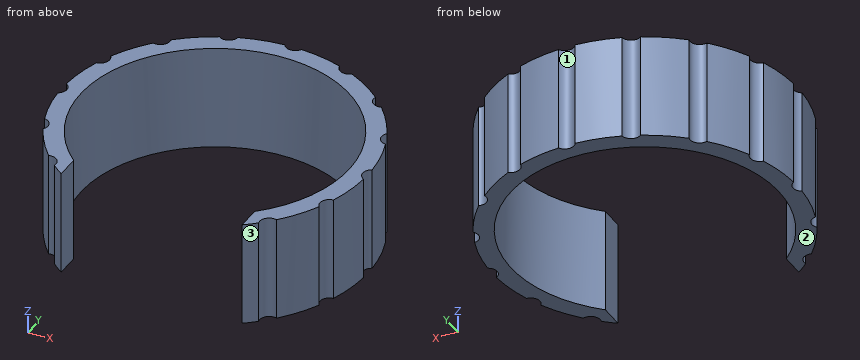
```python
from build123d import *

# Parameters (mm, degrees)
SKETCH3_W               = 140.131000148
SKETCH3_H               = 140
BOSS_EXTRUDE3_DEPTH     = 30
SKETCH3_7_OUTSIDE_W     = 182.199
SKETCH3_7_OUTSIDE_H     = 182.068
SKETCH3_7_OUTSIDE_W_2   = 140.131000148
SKETCH3_7_OUTSIDE_H_2   = 140
SKETCH3_7_OUTSIDE_R     = 32
CUT_EXTRUDE5_DEPTH      = 35
CUT_EXTRUDE6_DEPTH      = 10
CUT_EXTRUDE6_DEPTH_BACK = 5
SKETCH2_R               = 2.25
CUT_EXTRUDE8_DEPTH      = 207.479750358
CUT_EXTRUDE8_DEPTH_BACK = 207.479750358
SKETCH4_OUTSIDE_W       = 182.199
SKETCH4_OUTSIDE_H       = 182.068
SKETCH4_OUTSIDE_R       = 42.5
SKETCH5_OUTSIDE_W       = 111.78
SKETCH5_OUTSIDE_H       = 111.78
SKETCH5_OUTSIDE_R       = 36.5
CUT_EXTRUDE9_DEPTH      = 25
SKETCH2_3_R             = 2.25
CUT_EXTRUDE10_DEPTH     = 30
CUT_EXTRUDE14_DEPTH     = 25
SKETCH16_R              = 42.5
CUT_EXTRUDE15_DEPTH     = 5


with BuildPart() as part:
    # Sketch3 → Boss-Extrude3 (new body)
    with BuildSketch(Plane.XY):
        with Locations((-121.856065437, 0)):
            Rectangle(SKETCH3_W, SKETCH3_H)
    extrude(amount=BOSS_EXTRUDE3_DEPTH)

    # Sketch3_7 outside → Cut-Extrude5 (cut)
    # profile 1 of 2: a face of its own
    with BuildSketch(Plane.XY):
        with Locations((-121.8565, 0)):
            Rectangle(SKETCH3_7_OUTSIDE_W, SKETCH3_7_OUTSIDE_H)
        with Locations((-121.856065437, 0)):
            Rectangle(SKETCH3_7_OUTSIDE_W_2, SKETCH3_7_OUTSIDE_H_2, mode=Mode.SUBTRACT)
    # profile 2 of 2: a face of its own
    with BuildSketch(Plane.XY):
        with Locations(Location((-121.856065437, 0, 0), (0, 0, 180))):
            Circle(SKETCH3_7_OUTSIDE_R)
    extrude(amount=CUT_EXTRUDE5_DEPTH, mode=Mode.SUBTRACT)

    # Sketch2 → Cut-Extrude6 (cut, two sides: drawn at the far end of the back side and taken through both)
    with BuildSketch(Plane.XY.offset(-CUT_EXTRUDE6_DEPTH_BACK)):
        with Locations((-107.548664291, 34.645482469)):
            Circle(SKETCH2_R)
        with Locations((-95.38278871, 26.516504294)):
            Circle(SKETCH2_R)
        with Locations((-87.253810535, 14.350628714)):
            Circle(SKETCH2_R)
        with Locations((-84.399293004, 0)):
            Circle(SKETCH2_R)
        with Locations((-87.253810535, -14.350628714)):
            Circle(SKETCH2_R)
        with Locations((-95.38278871, -26.516504294)):
            Circle(SKETCH2_R)
        with Locations((-107.548664291, -34.645482469)):
            Circle(SKETCH2_R)
        with Locations((-121.899293004, -37.5)):
            Circle(SKETCH2_R)
        with Locations((-136.249921718, -34.645482469)):
            Circle(SKETCH2_R)
        with Locations((-148.415797299, -26.516504294)):
            Circle(SKETCH2_R)
        with Locations((-156.544775474, -14.350628714)):
            Circle(SKETCH2_R)
        with Locations((-159.399293004, 0)):
            Circle(SKETCH2_R)
        with Locations((-156.544775474, 14.350628714)):
            Circle(SKETCH2_R)
        with Locations((-148.415797299, 26.516504294)):
            Circle(SKETCH2_R)
        with Locations((-136.249921718, 34.645482469)):
            Circle(SKETCH2_R)
        with Locations((-121.899293004, 37.5)):
            Circle(SKETCH2_R)
    extrude(amount=CUT_EXTRUDE6_DEPTH + CUT_EXTRUDE6_DEPTH_BACK, mode=Mode.SUBTRACT)

    # Sketch4 outside → Cut-Extrude8 (cut, two sides: drawn at the far end of the back side and taken through both)
    with BuildSketch(Plane.XY.offset(30).offset(-CUT_EXTRUDE8_DEPTH_BACK)):
        with Locations((-121.8565, 0)):
            Rectangle(SKETCH4_OUTSIDE_W, SKETCH4_OUTSIDE_H)
        with Locations((-121.856065437, 0)):
            Circle(SKETCH4_OUTSIDE_R, mode=Mode.SUBTRACT)
    extrude(amount=CUT_EXTRUDE8_DEPTH + CUT_EXTRUDE8_DEPTH_BACK, mode=Mode.SUBTRACT)

    # Sketch5 outside → Cut-Extrude9 (cut)
    with BuildSketch(Plane.XY.offset(30)):
        with Locations((-121.856, 0)):
            Rectangle(SKETCH5_OUTSIDE_W, SKETCH5_OUTSIDE_H)
        with Locations((-121.856065437, 0)):
            Circle(SKETCH5_OUTSIDE_R, mode=Mode.SUBTRACT)
    extrude(amount=-CUT_EXTRUDE9_DEPTH, mode=Mode.SUBTRACT)

    # Sketch2_3 → Cut-Extrude10 (cut)
    with BuildSketch(Plane.XY):
        with Locations(Location((-107.548664291, 34.645482469, 0), (0, 0, 310.084812014))):
            Circle(SKETCH2_3_R)
        with Locations(Location((-95.38278871, 26.516504294, 0), (0, 0, 287.961507123))):
            Circle(SKETCH2_3_R)
        with Locations(Location((-87.253810535, 14.350628714, 0), (0, 0, 265.700727885))):
            Circle(SKETCH2_3_R)
        with Locations(Location((-84.399293004, 0, 0), (0, 0, 116.73315475))):
            Circle(SKETCH2_3_R)
        with Locations(Location((-87.253810535, -14.350628714, 0), (0, 0, 94.299272115))):
            Circle(SKETCH2_3_R)
        with Locations(Location((-95.38278871, -26.516504294, 0), (0, 0, 72.038492877))):
            Circle(SKETCH2_3_R)
        with Locations(Location((-107.548664291, -34.645482469, 0), (0, 0, 49.915187986))):
            Circle(SKETCH2_3_R)
        with Locations(Location((-121.899293004, -37.5, 0), (0, 0, 27.872824405))):
            Circle(SKETCH2_3_R)
        with Locations(Location((-136.249921718, -34.645482469, 0), (0, 0, 5.842100852))):
            Circle(SKETCH2_3_R)
        with Locations(Location((-148.415797299, -26.516504294, 0), (0, 0, 343.751257801))):
            Circle(SKETCH2_3_R)
        with Locations(Location((-156.544775474, -14.350628714, 0), (0, 0, 321.537161827))):
            Circle(SKETCH2_3_R)
        with Locations(Location((-159.399293004, 0, 0), (0, 0, 60.844584247))):
            Circle(SKETCH2_3_R)
        with Locations(Location((-156.544775474, 14.350628714, 0), (0, 0, 38.462838173))):
            Circle(SKETCH2_3_R)
        with Locations(Location((-148.415797299, 26.516504294, 0), (0, 0, 16.248742199))):
            Circle(SKETCH2_3_R)
        with Locations(Location((-136.249921718, 34.645482469, 0), (0, 0, 354.157899148))):
            Circle(SKETCH2_3_R)
        with Locations(Location((-121.899293004, 37.5, 0), (0, 0, 332.127175595))):
            Circle(SKETCH2_3_R)
    extrude(amount=CUT_EXTRUDE10_DEPTH, mode=Mode.SUBTRACT)

    # Sketch15 → Cut-Extrude14 (cut)
    with BuildSketch(Plane.XY.offset(30)):
        with BuildLine():
            Line((-143.464225434, -37.475141345), (-143.420997866, 0.024858655))
            ThreePointArc((-143.420997866, 0.024858655), (-121.831206782, 21.564932429), (-100.291133008, -0.024858655))
            Line((-100.291133008, -0.024858655), (-100.334360575, -37.524858655))
            ThreePointArc((-100.334360575, -37.524858655), (-121.92415166, -59.064932429), (-143.464225434, -37.475141345))
        make_face()
    extrude(amount=-CUT_EXTRUDE14_DEPTH, mode=Mode.SUBTRACT)

    # Sketch16 → Cut-Extrude15 (cut)
    with BuildSketch(Plane(origin=(0, 0, 0), x_dir=(-1, 0, 0), z_dir=(0, 0, -1))):
        with Locations((121.856065437, 0)):
            Circle(SKETCH16_R)
    extrude(amount=-CUT_EXTRUDE15_DEPTH, mode=Mode.SUBTRACT)


solid = part.part
```
Work out the finished part from the listing and answer in its coordinate system (mm). Face numbers are marked on the shaded views. Round coordinates to 2 decimals unless told otherwise and drop trailing zeros. Order: outer loops, then holes, each group sorted by start corner. A loop starts at its lowest first (then second) coordinate and runs counter-clockwise, first axis right, second up.
Q1. A cutting plane is placed at D-D, the plane x = -108. Determine the outline of the cut face in (y, z), then the cut area to 3 significant figures.
Solution:
outline: (28.84, 5) - (32.44, 5) - (32.44, 30) - (28.84, 30) - close
area: 89.9 mm2
Q2. Find the intervals of material crossed by line 1 along X through (y, z) = (0, 13.75); line 2 along X through (y, z) = (-20.5, 10); line 3 along Y through (x, z) = (-132, 22.5), in increasing order.
Solution:
line 1: x = -157.15 to -153.86, -89.86 to -86.65
line 2: x = -152.06 to -146.43, -97.28 to -91.66
line 3: y = 30.35 to 35.06
Q3. A cutting plane is placed at C-C, the plane y = 22. Determine the outline of the cut face in (x, z), then the cut area to 3 significant figures.
Solution:
outline: (-150.98, 5) - (-145.09, 5) - (-145.09, 30) - (-150.98, 30) - close; (-98.62, 5) - (-92.73, 5) - (-92.73, 30) - (-98.62, 30) - close
area: 294 mm2
Q4. The mould has two halves that part along X. Classify the marked faces 1, 2 and 3: pulls with the +X half, pulls with the -X half, needs draft (parallel to the pull), parting line crosses it, or undercut.
Solution:
face 1: undercut
face 2: needs draft
face 3: pulls with the +X half
Q5. A cutting plane is placed at A-A, the plane y = 0. Determine the outline of the cut face in (x, z).
Solution:
outline: (-157.15, 5) - (-153.86, 5) - (-153.86, 30) - (-157.15, 30) - close; (-89.86, 5) - (-86.65, 5) - (-86.65, 30) - (-89.86, 30) - close
Q6. Given pin 1 Ø8 at (y, z) = (20.5, 25.5) entering from -X; pin 2 Ø2 at (y, z) = (5.5, 22.5) entering from -X; pin 3 Ø3 at (x, z) = (-122, 11.5) entering from +Y, each flat-ended and moving along its own axis, determine where each tip first touches the part or whether it passes through.
Solution:
pin 1: stops at x = -154.41
pin 2: stops at x = -158.08
pin 3: stops at y = 35.92
